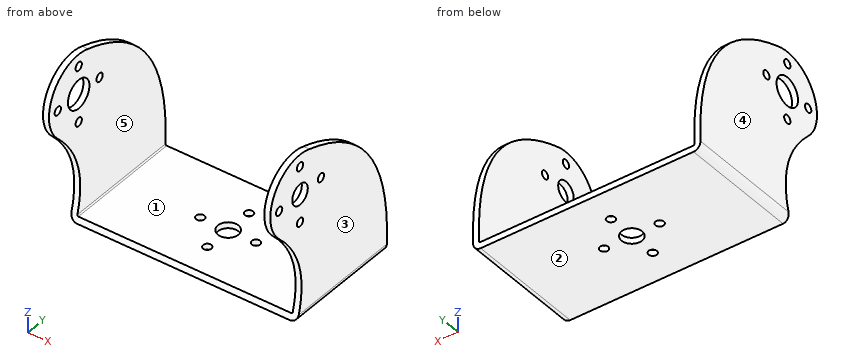
Autodesk Inventor part; units mm, degrees
ref_plane "YZ Plane" through (0, 0, 0) normal (1, 0, 0) x (0, 1, 0)
ref_plane "XZ Plane" through (0, 0, 0) normal (0, 1, 0) x (-1, 0, 0)
ref_plane "XY Plane" through (0, 0, 0) normal (0, 0, 1) x (1, 0, 0)
sketch "Sketch1" plane through (0, 0, 0) normal (0, 0, 1) x (1, 0, 0)
  line L0 (-28.59, -25) -> (28.59, -25)
  line L1 (28.59, -25) -> (28.59, 25)
  line L2 (28.59, 25) -> (-28.59, 25)
  line L3 (-28.59, 25) -> (-28.59, -25)
  line L4 (-28.59, -25) -> (28.59, 25) construction
  line L5 (28.59, -25) -> (-28.59, 25) construction
  point P0 (0, 0)
  dimension "d0" = 57.18
  dimension "d1" = 50
extrude "Plate1" add sketch "Sketch1" along normal blind 1.5
sketch "Sketch2" plane through (-27.09, -25, 0) normal (-1, 0, 0) x (0, -1, 0)
  line L0 (-50, 0) -> (0, 0)
  line L1 (0, 0) -> (0, 45)
  line L2 (0, 45) -> (-50, 45)
  line L3 (-50, 45) -> (-50, 0)
edge flange "Flange1" height 45 angle 90 thickness 1.5 bend radius 0.31 thickness toward (-1, 0, 0) relief tear relief width 1.5 relief depth 0.75 corner gap 0.31 corner form 0 edges at (-28.59, 0, 1.5) (28.59, 0, 1.5) wall of the first edge with corners at (-27.09, 25, 0) (-27.09, -25, 0) (-27.09, -25, 45) (-27.09, 25, 45)
bend "Bend1"
corner "Corner1"
sketch "Sketch17" plane through (0, 0, 1.5) normal (0, 0, 1) x (1, 0, 0)
  circle A0 centre (0, 7) radius 0.7835
  circle A1 centre (7, 0) radius 0.7835
  circle A2 centre (0, -7) radius 0.7835
  circle A3 centre (-7, 0) radius 0.7835
  point P0 (0, 0)
hole "Hole7" at (0, 7, 1.5) at (7, 0, 1.5) at (0, -7, 1.5) at (-7, 0, 1.5) direction (0, 0, -1) diameter 2.1 depth 1.5
sketch "Sketch26" plane through (28.59, -25, 45) normal (1, 0, 0) x (0, 0, -1)
  arc A0 (3.5502, 14.1468) -> (20.0473, 3.9617) centre (13, 11) ccw
  line L0 (45, 50) -> (45, 0)
  spline S0 degree 2 poles (3.5502, 14.1468) (11.7245, 42.1837) (45, 40) knots 0 0 0 1 1 1
  spline S1 degree 2 poles (20.0473, 3.9617) (31.1315, 14.9193) (45, 10) knots 0 0 0 1 1 1
  line L1 (45, 10) -> (45, 40)
  line L2 (0, 0) -> (45, 0)
  line L3 (45, 0) -> (45, 50)
  line L4 (45, 50) -> (0, 50)
  line L5 (0, 50) -> (0, 0)
  point P0 (45, 25)
  point P1 (45, 25)
  point P2 (17.1562, 34.0829)
  point P3 (32.0366, 10.9995)
  dimension "d143" = 19.92
  dimension "d144" = 32
  dimension "d145" = 14
  dimension "d160" = 15
  dimension "d161" = 15
  dimension "d162" = 7.0473
  dimension "d163" = 9.4498
  dimension "d164" = 19.0366
  dimension "d165" = 7.0378
  dimension "d166" = 13.606
  dimension "d167" = 19.9361
extrude "Cut8" cut sketch "Sketch26" against normal blind 57.18 contours A0 S1 L0 L2 L5 L4 S0
sketch "Sketch27" plane through (-28.59, -14.4222, 1.81) normal (-1, 0, 0) x (0, 0, 1)
  circle A0 centre (23.12, 0.4222) radius 0.7835
  circle A1 centre (30.12, -6.5778) radius 0.7835
  circle A2 centre (30.12, 7.4222) radius 0.7835
  circle A3 centre (37.12, 0.4222) radius 0.7835
  point P0 (-1.81, 14.4222)
hole "Hole15" at (-28.59, -14, 24.93) at (-28.59, -7, 31.93) at (-28.59, -21, 31.93) at (-28.59, -14, 38.93) direction (1, 0, 0) diameter 2.1 depth 1.5
sketch "Sketch28" plane through (28.59, -14.4222, 1.81) normal (1, 0, 0) x (0, 0, -1)
  circle A0 centre (-23.12, 0.4222) radius 0.7835
  circle A1 centre (-30.12, -6.5778) radius 0.7835
  circle A2 centre (-37.12, 0.4222) radius 0.7835
  circle A3 centre (-30.12, 7.4222) radius 0.7835
  point P0 (1.81, 14.4222)
hole "Hole16" at (28.59, -14, 24.93) at (28.59, -7, 31.93) at (28.59, -21, 31.93) at (28.59, -14, 38.93) direction (-1, 0, 0) diameter 2.1 depth 1.5
sketch "Sketch29" plane through (-28.59, -14.4222, 1.81) normal (-1, 0, 0) x (0, 0, 1)
  circle A0 centre (30.12, 0.4222) radius 1.2295
  point P0 (-1.81, 14.4222)
hole "Hole17" at (-28.59, -14, 31.93) direction (1, 0, 0) diameter 7.2 depth 1.5
sketch "Sketch30" plane through (28.59, -14.4222, 1.81) normal (1, 0, 0) x (0, 0, -1)
  circle A0 centre (-30.12, 0.4222) radius 1.75
  point P0 (1.81, 14.4222)
hole "Hole18" at (28.59, -14, 31.93) direction (-1, 0, 0) diameter 5.2 depth 1.5
sketch "Sketch31" plane through (0, 0, 1.5) normal (0, 0, 1) x (1, 0, 0)
  circle A0 centre (0, 0) radius 1.75
  point P0 (0, 0)
hole "Hole19" at (0, 0, 1.5) direction (0, 0, -1) diameter 5.2 depth 1.5
equation "\"d90\" = Thickness"
equation "\"d2\" = Thickness"
equation "\"d3\" = BendReliefWidth"
equation "\"d4\" = BendReliefDepth"
equation "\"d5\" = MinimumRemnant"
equation "\"d6\" = TransitionRadius"
equation "\"d9\" = BendRadius"
equation "\"d10\" = CornerReliefSize"
equation "\"d11\" = GapSize"
equation "\"d12\" = JacobiRadiusSize"
equation "\"BendReliefWidth\" = Thickness"
equation "\"BendReliefDepth\" = 0.5 * Thickness"
equation "\"CornerReliefSize\" = 4 * Thickness"
equation "\"MinimumRemnant\" = 2 * Thickness"
equation "\"TransitionRadius\" = BendRadius"
equation "\"JacobiRadiusSize\" = BendRadius"
equation "\"GapSize\" = Thickness"
properties part number "axis_15_bottom_frame" material "Aluminum 6061-AHC"
Verification items for the finished model (mm, model axes). Face numbers are marked on the shaded views. A direction names the side the tool comes from. Coordinates: 2 decimals unless noted, no trailing zeros. Use CSV: the item, a comma, the result in double quotes.
Q1. Mould release check, pull along X, two halves, no side actions. Record for the marked faces 3, 4 and 5: pulls with the +X half, pulls with the -X half, needs draft (parallel to the pull), parting line crosses it, or undercut.
Computed values:
face 3,"pulls with the +X half"
face 4,"pulls with the -X half"
face 5,"undercut"
Q2. Go/stop test with flat-tipped pins: P1, Ø2.5, axis at x = -7, y = 0, coming from the +Z side; P2, Ø1.9, axis at y = -21, z = 31.93, coming from the +X side; P3, Ø6, axis at y = -14, z = 31.93, coming from the -X side. Record where each tip stops, or that it passes through.
Computed values:
P1,"z = 1.5"
P2,"through"
P3,"x = 27.09"
Q3. Set-up check for the marked faces 1 and 2: record each of +Z, -Z, +X, -X, +Y, -Y from which the full face is reachable in a straight line by a thin tool's end or side.
Computed values:
face 1,"+Z, +Y, -Y"
face 2,"-Z, +X, -X, +Y, -Y"
Q4. Thickness scan on line 1 along X through (y, z) = (-4, 5); line 2 along Y through (x, z) = (0, 0.5); line 3 along Y through (x, z) = (27.9, 31.93). Record the ranges inside material, lowest first. Write a range as [from, to].
Computed values:
line 1,"[-28.59, -27.09], [27.09, 28.59]"
line 2,"[-14.83, -8.05], [-5.95, -2.6], [2.6, 5.95], [8.05, 15.03]"
line 3,"[-23.96, -22.05], [-19.95, -16.6], [-11.4, -8.05], [-5.95, 5.79]"
Q5. Section check A-A, the plane y = 0. State how many separate pieces and enclosed holes the cut face has, and give its area (3 significant figures).
Computed values:
separate pieces,"4"
enclosed holes,"0"
area,"176 mm²"
